```python
from build123d import *

# Parameters (mm, degrees)
F0_W          = 7
F0_H          = 20
F2_DEPTH      = 10
F2_DEPTH_BACK = 10
F1_R          = 8.875
F3_DEPTH      = 25
F3_DEPTH_BACK = 25
F5_DEPTH      = 1.5
F7_DEPTH      = 1.5
F8_SIZE       = 0.5


with BuildPart() as f2:
    # F0 (on Right) → F2 (new body, two sides)
    with BuildSketch(Plane.YZ) as f2_sk:
        Polygon((5, 11.5), (3.5, 11.5), (-3.5, 11.5), (-5, 11.5), (-5, -11.5), (5, -11.5), align=None)
        Rectangle(F0_W, F0_H, mode=Mode.SUBTRACT)
        Polygon((-3.5, 11.5), (3.5, 11.5), (5, 11.5), (5, 13), (-3.5, 13), align=None)
    extrude(amount=F2_DEPTH)
    extrude(f2_sk.sketch, amount=-F2_DEPTH_BACK)

    # F1 (on Front) → F3 (cut, two sides)
    with BuildSketch(Plane.XZ) as f3_sk:
        Circle(F1_R)
    extrude(amount=-F3_DEPTH, mode=Mode.SUBTRACT)
    extrude(f3_sk.sketch, amount=F3_DEPTH_BACK, mode=Mode.SUBTRACT)

    # F4 (on face) → F5 (cut)
    with BuildSketch(Plane.XY.offset(13)):
        with BuildLine():
            ThreePointArc((0, -3.5), (-6.220128616, -1.4488224541), (-10, 3.9))
            Line((-10, 3.9), (-10, -3.5))
            Line((-10, -3.5), (0, -3.5))
        make_face()
        with BuildLine():
            ThreePointArc((10, 3.9), (6.220128616, -1.4488224541), (0, -3.5))
            Line((0, -3.5), (10, -3.5))
            Line((10, -3.5), (10, 3.9))
        make_face()
    extrude(amount=-F5_DEPTH, mode=Mode.SUBTRACT)

    # F6 (on face) → F7 (cut)
    with BuildSketch(Plane(origin=(0, 0, 10), x_dir=(1, 0, 0), z_dir=(0, 0, -1))):
        with BuildLine():
            ThreePointArc((10, 3.5), (0, -0.4807811985), (-10, 3.5))
            Line((-10, 3.5), (-10, -3.5))
            Line((-10, -3.5), (10, -3.5))
            Line((10, -3.5), (10, 3.5))
        make_face()
    extrude(amount=-F7_DEPTH, mode=Mode.SUBTRACT)

    # F8
    f8_edges = [f2.edges().sort_by_distance(p)[0] for p in [
        (-8.875, -5, 0),
        (-8.875, 5, 0),
    ]]
    chamfer(f8_edges, length=F8_SIZE)


solid = f2.part
```
Geometry: final body of the model. Coordinates: model frame, mm. A direction names the side the tool comes from. Round coordinates to 2 decimals unless told otherwise and drop trailing zeros. Loops run counter-clockwise (first coordinate to the right, second up) from the corner with the lowest first, then second, coordinate; pieces in that order, holes last.
Item 1: Line query: L1, parallel to Z at x = 8.5, y = 1; L2, parallel to Z at x = 0, y = 3.7 (3 decimals); L3, parallel to Y at x = 3, z = -9.25. Output: solid intervals per line, ascending.
Checked values:
L1: z = -11.5 to -10, 11.5 to 13
L2: z = -11.5 to -8.875, 8.875 to 13
L3: y = -5 to -3.5, 3.5 to 5
Item 2: Mould query, pull axis X, two halves, no side actions, for faces 5 (the cylindrical face through (-1.924, -3.993, -8.664)), 6 (the flat face through (0, 0, -11.5)), 7 (the flat face through (-10, 4, 0)), 8 (the cylindrical face through (-1.924, 3.993, -8.664)). Classes: released by +X, released by -X, zero draft, split by the parting line, or undercut.
Checked values:
face 5: undercut
face 6: zero draft
face 7: released by -X
face 8: undercut
Item 3: Section A-A, the plane z = 0. Output: boundary loops of the cut face in (x, y) (3 decimals), plus the area to 3 significant figures.
Checked values:
outline: (-10, -5) - (-9.375, -5) - (-8.875, -4.5) - (-8.875, -3.5) - (-10, -3.5) - close; (-10, 3.5) - (-8.875, 3.5) - (-8.875, 4.5) - (-9.375, 5) - (-10, 5) - close; (8.875, -4.5) - (9.375, -5) - (10, -5) - (10, -3.5) - (8.875, -3.5) - close; (8.875, 3.5) - (10, 3.5) - (10, 5) - (9.375, 5) - (8.875, 4.5) - close
area: 6.25 mm2
Item 4: Section D-D, the plane y = 1.5. Output: boundary loops of the cut face in (x, z).
Checked values:
outline: (-10, -11.5) - (10, -11.5) - (10, -10) - (-10, -10) - close; (-8.92, 11.5) - (8.92, 11.5) - (8.92, 13) - (-8.92, 13) - close
Item 5: Section C-C, the plane x = 7.25. State how many separate pieces and enclosed holes the cut face has, plus the area to 3 significant figures.
Checked values:
separate pieces: 3
enclosed holes: 0
area: 59.4 mm2
Item 6: Reachability of faces 1 (the flat face through (10, 4, 0)), 2 (the flat face through (0, -4, 11.5)), 3 (the flat face through (0, 0, -10)), 4 (the cylindrical face through (0.15, 0.48, 10.74)) from +Z, -Z, +X, -X, +Y, -Y: full face, straight path, thin tool, end or side. Return the list, or none.
Checked values:
face 1: +Z, -Z, +X, +Y, -Y
face 2: +Z, -Y
face 3: +X, -X
face 4: none
Item 7: Contact query for flat-ended pins moving along their axis: P1, Ø6, axis at x = 3.5, z = 5, coming from the -Y side; P2, Ø10, axis at x = -1.5, z = -2.5, coming from the +Y side. Output: stop coordinate, or through.
Checked values:
P1: stops at y = -4.73
P2: passes through
Item 8: Section B-B, the plane y = -2. Output: boundary loops of the cut face in (x, z).
Checked values:
outline: (-10, -11.5) - (10, -11.5) - (10, -10) - (-10, -10) - close; (-8.13, 10) - (8.13, 10) - (8.13, 11.5) - (5.4, 11.5) - (5.4, 13) - (-5.4, 13) - (-5.4, 11.5) - (-8.13, 11.5) - close
